For this review, use the dimensioned drawing (mm, ordinates from the lowest corner) and the shaded views. A direction names the side the tool comes from. Round coordinates to 2 decimals unless told otherwise and drop trailing zeros. Write each loop counter-clockwise with the first axis right and the second up, starting at its lowest first coordinate (ties: lowest second). Pieces come first, ordered by that corner, then holes. Notation, with made-up numbers: (50.5, 78) -> (109.5, 78) arc R11 ccw to (109.5, 91) -> close; hole circle Ø3 at (-13, 33.5). An arc over 180 degrees is marked (long way). Write each question's results on one line, items separated by ' | '. Start each with the question number.
Item 1: Tool access review of the marked faces 4, 5 and 6: name each direction out of +Z, -Z, +X, -X, +Y, -Y from which nothing blocks a thin tool from reaching the whole face with its end or side.
Item 2: Add section C-C (y = 3). State the section outline as (x, z) points, plus the area to 3 significant figures.
Item 3: The part is to be moulded in two halves that separate along X. For the marked faces 1, 2 and 3, say which applies: +X half, -X half, draft (parallel to the pull), parting line (faces both ways), or undercut.
Item 4: Clearance check with flat-ended pins moving along their axes: pin 1 (6.5 mm diameter, centred on x = 10, z = 49, fed in from +Y); pin 2 (3 mm diameter, centred on x = 15, z = 7.5, fed in from -Y); pin 3 (1.5 mm diameter, centred on y = 9.5, z = 9, fed in from -X); pin 4 (11.5 mm diameter, centred on x = 10.5, z = 13.5, fed in from -Y). State where each tip first meets the part, or that it passes through.
Item 5: Add section D-D (x = 23). State the section outline as (y, z) points, plus the area to 3 significant figures.
Item 6: Add section B-B (z = 49). State the section outline as (x, y) points.
Item 7: To check wall thickness, follow line 1 along Z through (x, y) = (30, 3.2); line 2 along Z through (x, y) = (15, 13.6); line 3 along Y through (x, z) = (21.5, 28). State the ranges of each line that lie inside material, in increasing order.
Item 8: Add section A-A (x = 15). State the section outline as (y, z) points, plus the area to 3 significant figures.
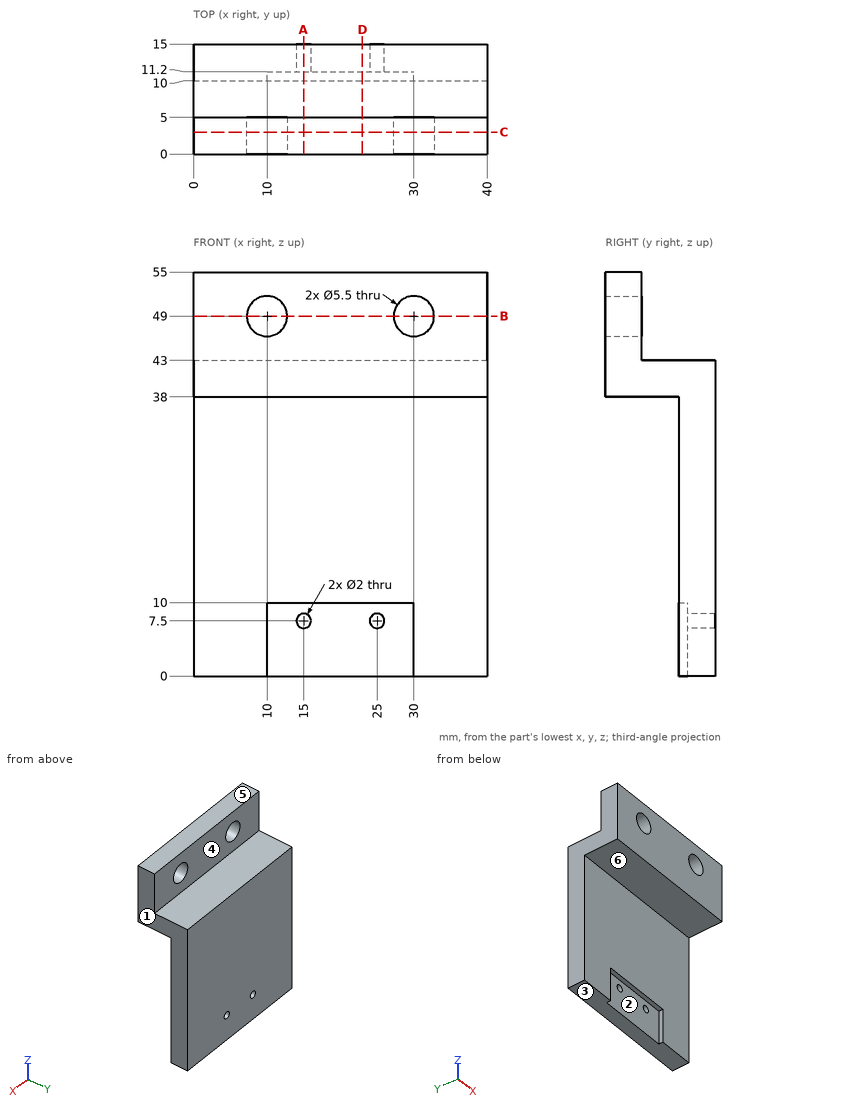
Responses:
1) face 4: +Z, +X, -X, +Y | face 5: +Z, +X, -X, +Y, -Y | face 6: -Z, +X, -X, -Y
2) outline: (0, 38) -> (40, 38) -> (40, 55) -> (0, 55) -> close; hole circle Ø5.5 at (10, 49); hole circle Ø5.5 at (30, 49) | area: 632 mm^2
3) face 1: +X half | face 2: undercut | face 3: draft
4) pin 1: stops at y = 5 | pin 2: stops at y = 11.2 | pin 3: stops at x = 0 | pin 4: stops at y = 10
5) outline: (0, 38) -> (10, 38) -> (10, 10) -> (11.2, 10) -> (11.2, 0) -> (15, 0) -> (15, 43) -> (5, 43) -> (5, 55) -> (0, 55) -> close | area: 313 mm^2
6) outline: (0, 0) -> (7.25, 0) -> (7.25, 5) -> (0, 5) -> close; (12.75, 0) -> (27.25, 0) -> (27.25, 5) -> (12.75, 5) -> close; (32.75, 0) -> (40, 0) -> (40, 5) -> (32.75, 5) -> close
7) line 1: z = 38 to 46.25, 51.75 to 55 | line 2: z = 0 to 6.5, 8.5 to 43 | line 3: y = 10 to 15
8) outline: (0, 38) -> (10, 38) -> (10, 10) -> (11.2, 10) -> (11.2, 8.5) -> (15, 8.5) -> (15, 43) -> (5, 43) -> (5, 55) -> (0, 55) -> close; (11.2, 0) -> (15, 0) -> (15, 6.5) -> (11.2, 6.5) -> close | area: 305 mm^2
